Print and shaded views of the part. All mm, measured from the part's lowest x, y and z. A direction names the side the tool comes from. Round coordinates to 2 decimals unless told otherwise and drop trailing zeros. Loops run counter-clockwise (first coordinate to the right, second up) from the corner with the lowest first, then second, coordinate; pieces in that order, holes last. Notation, with made-up numbers: (56, 7) - (74, 7) arc R17 ccw to (74, 25) - close; hole circle Ø7 at (52, 45.25). An arc over 180 degrees is marked (long way). Use one line per item in the form item = value.
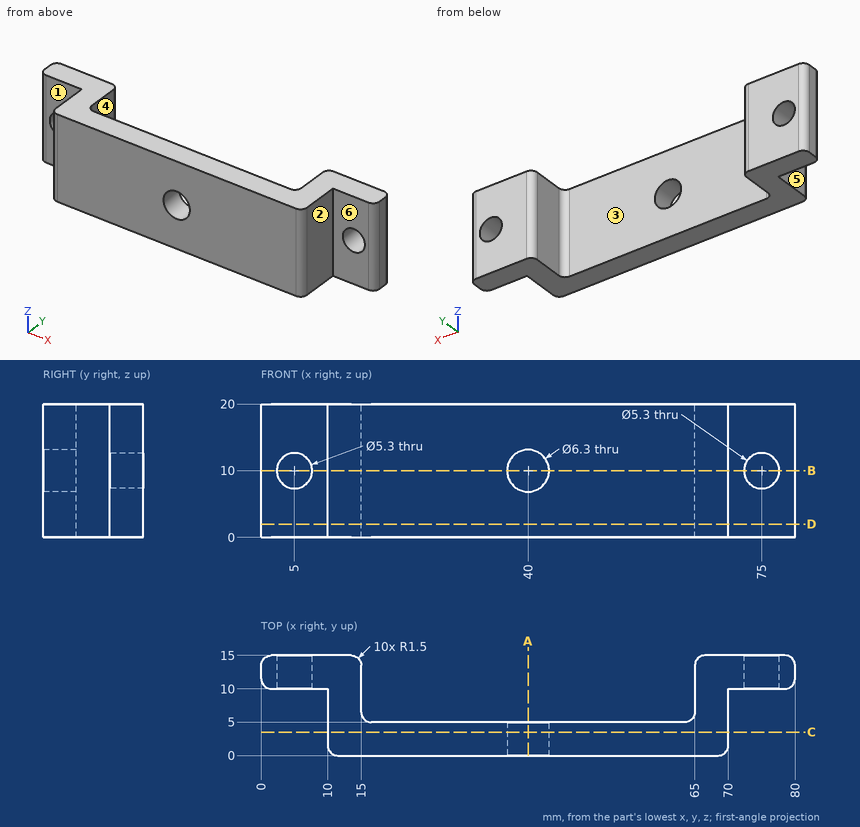
1. Pull direction X, two halves, no side cores. Call the marked faces 4, 5 and 6: +X half, -X half, draft (parallel to the pull), parting line (faces both ways), or undercut.
Geometry check:
face_4 = undercut
face_5 = -X half
face_6 = draft
2. Cut at B-B, the plane z = 10. Give the number of separate pieces and of enclosed holes in the cut face, plus the area to 3 significant figures.
Geometry check:
separate_pieces = 4
enclosed_holes = 0
area = 413 mm^2
3. Tool access for the marked faces 1, 2 and 3: list every direction of +Z, -Z, +X, -X, +Y, -Y with a clear straight run to the whole face (end or side of a thin tool).
Geometry check:
face_1 = +Z, -Z, -X, -Y
face_2 = +Z, -Z, +X, -Y
face_3 = +Z, -Z, +Y
4. Wall check: probe 1 along X at (y, z) = (12.25, 9.75); probe 2 along Z at (x, y) = (5, 13); probe 3 along Z at (x, y) = (40, 3.8). Give the ranges that are in metal, low to high.
Geometry check:
probe_1 = 0 to 2.36, 7.64 to 15, 65 to 72.36, 77.64 to 80
probe_2 = 0 to 7.35, 12.65 to 20
probe_3 = 0 to 6.85, 13.15 to 20
5. Cut at D-D, the plane z = 2. Give the cut face in (x, y), plus the area to 3 significant figures.
Geometry check:
outline = (0, 11.5) arc R1.5 ccw to (1.5, 10) - (10, 10) - (10, 1.5) arc R1.5 ccw to (11.5, 0) - (68.5, 0) arc R1.5 ccw to (70, 1.5) - (70, 10) - (78.5, 10) arc R1.5 ccw to (80, 11.5) - (80, 13.5) arc R1.5 ccw to (78.5, 15) - (66.5, 15) arc R1.5 ccw to (65, 13.5) - (65, 6.5) arc R1.5 cw to (63.5, 5) - (16.5, 5) arc R1.5 cw to (15, 6.5) - (15, 13.5) arc R1.5 ccw to (13.5, 15) - (1.5, 15) arc R1.5 ccw to (0, 13.5) - close
area = 497 mm^2
6. Cut at A-A, the plane x = 40. Give the cut face in (y, z).
Geometry check:
outline = (0, 0) - (5, 0) - (5, 6.85) - (0, 6.85) - close; (0, 13.15) - (5, 13.15) - (5, 20) - (0, 20) - close
7. Cut at C-C, the plane y = 3.5. Give the cut face in (x, z).
Geometry check:
outline = (10, 0) - (70, 0) - (70, 20) - (10, 20) - close; hole circle Ø6.3 at (40, 10)
8. Flat gauge pins, fed straight in: pin 1 (4 mm diameter, centred on y = 6, z = 7.5, fed in from +X); pin 2 (7 mm diameter, centred on x = 7.5, z = 13.5, fed in from -Y); pin 3 (6 mm diameter, centred on x = 5, z = 10, fed in from -Y); pin 4 (4 mm diameter, centred on x = 40, z = 10, fed in from +Y). Where does each tip first touch, or does it go through?
Geometry check:
pin_1 = 70
pin_2 = 0.09
pin_3 = 10
pin_4 = through
